Read the model definition and answer for the solid it produces. Units are mm, in the model's axes. Face numbers are marked on the shaded views. A direction names the side the tool comes from. Give positions to 0.01 mm unless a question says otherwise; leave off trailing zeros. Order: outer loops, then holes, each group sorted by start corner. A loop starts at its lowest first (then second) coordinate and runs counter-clockwise, first axis right, second up. Notation, with made-up numbers: (40.5, -18) - (55.5, -18) arc R30 ccw to (55.5, 12) - close; hole circle Ø4 at (-20.75, 79). An arc over 180 degrees is marked (long way). One line per item, written item: value. Start each with the question number.
```python
from build123d import *

# Parameters (mm, degrees)
F0_W     = 105
F0_H     = 90
F0_W_2   = 90
F0_H_2   = 80
F1_DEPTH = 15.3
F2_R     = 5.069848481
F0_W_3   = 69
F0_H_3   = 58
F3_DEPTH = 5.5
F4_DEPTH = 11.8
F5_R     = 4.8284271247


with BuildPart() as f1:
    # F0 (on Top) → F1 (new body, symmetric)
    with BuildSketch(Plane.XY):
        Rectangle(F0_W, F0_H)
        Rectangle(F0_W_2, F0_H_2, mode=Mode.SUBTRACT)
    extrude(amount=F1_DEPTH, both=True)

    # F2
    f2_edges = [f1.edges().sort_by_distance(p)[0] for p in [
        (52.5, -45, 0),
        (-52.5, -45, 0),
        (-52.5, 45, 0),
        (52.5, 45, 0),
    ]]
    fillet(f2_edges, radius=F2_R)

    # F0 (on Top) → F3 (join)
    with BuildSketch(Plane.XY):
        Rectangle(F0_W_2, F0_H_2)
        Rectangle(F0_W_3, F0_H_3, mode=Mode.SUBTRACT)
    extrude(amount=F3_DEPTH)

    # F0 (on Top) → F4 (join)
    with BuildSketch(Plane.XY):
        Rectangle(F0_W_3, F0_H_3)
    extrude(amount=F4_DEPTH)

    # F5
    f5_edges = [f1.edges().sort_by_distance(p)[0] for p in [
        (34.5, -29, 8.65),
        (34.5, 29, 8.65),
        (-34.5, 29, 8.65),
        (-34.5, -29, 8.65),
    ]]
    fillet(f5_edges, radius=F5_R)


solid = f1.part
```
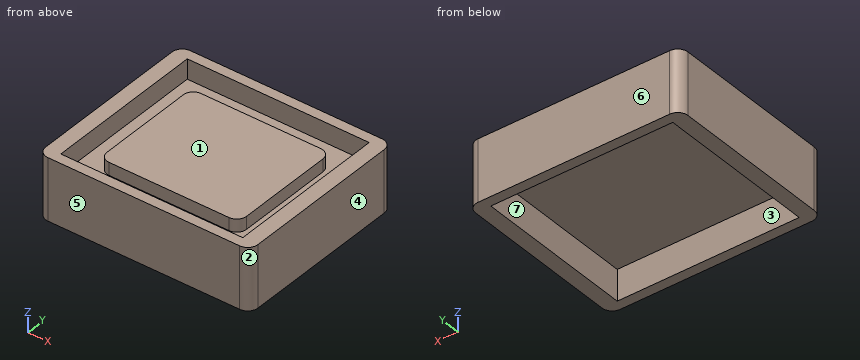
1) Section A-A on z = 9.5 is taken. Write down the section's boundary in (x, y), plus the area to 3 significant figures.
2) Section C-C on y = 7.5 is taken. Write down the section's boundary in (x, z), plus the area to 3 significant figures.
3) Section D-D on x = -23 is taken. Write down the section's boundary in (y, z), plus the area to 3 significant figures.
4) Find the intervals of material crossed by probe 1 along Y at (x, z) = (-10.5, 10.5); probe 2 along X at (y, z) = (-12.5, -10.5); probe 3 along Y at (x, z) = (32, 10.5), in increasing order. Write a range as from..to.
5) For the marked faces 1, 2 and 3, determine the directions among +Z, -Z, +X, -X, +Y, -Y from which every point of the face is accessible in a straight line to the end or side of a thin tool.
6) Each of these flat-tipped pins is pushed along its axis until it touches: pin 1 (1.5 mm diameter, centred on x = -9.5, y = 35, fed in from +Z); pin 2 (12 mm diameter, centred on x = -25.5, y = -27.5, fed in from -Z); pin 3 (17.5 mm diameter, centred on x = -15, y = -3, fed in from +Z). Where does it stop, or does it pass through?
7) Section B-B on x = 40 is taken. Write down the section's boundary in (y, z).
8) The mould has two halves that part along Y. Classify the marked faces 4, 5, 6 and 7: +Y half, -Y half, draft (parallel to the pull), parting line (faces both ways), or undercut.
Solved:
1. outline: (-52.5, -39.93) arc R5.07 ccw to (-47.43, -45) - (47.43, -45) arc R5.07 ccw to (52.5, -39.93) - (52.5, 39.93) arc R5.07 ccw to (47.43, 45) - (-47.43, 45) arc R5.07 ccw to (-52.5, 39.93) - close; (-34.5, -24.17) arc R4.83 ccw to (-29.67, -29) - (29.67, -29) arc R4.83 ccw to (34.5, -24.17) - (34.5, 24.17) arc R4.83 ccw to (29.67, 29) - (-29.67, 29) arc R4.83 ccw to (-34.5, 24.17) - close; hole (-45, -40) - (45, -40) - (45, 40) - (-45, 40) - close
1. area: 6,210 mm2
2. outline: (-52.5, -15.3) - (-45, -15.3) - (-45, 0) - (45, 0) - (45, -15.3) - (52.5, -15.3) - (52.5, 15.3) - (45, 15.3) - (45, 5.5) - (34.5, 5.5) - (34.5, 11.8) - (-34.5, 11.8) - (-34.5, 5.5) - (-45, 5.5) - (-45, 15.3) - (-52.5, 15.3) - close
2. area: 1,390 mm2
3. outline: (-45, -15.3) - (-40, -15.3) - (-40, 0) - (40, 0) - (40, -15.3) - (45, -15.3) - (45, 15.3) - (40, 15.3) - (40, 5.5) - (29, 5.5) - (29, 11.8) - (-29, 11.8) - (-29, 5.5) - (-40, 5.5) - (-40, 15.3) - (-45, 15.3) - close
3. area: 1,110 mm2
4. probe 1: y = -45..-40, -29..29, 40..45
4. probe 2: x = -52.5..-45, 45..52.5
4. probe 3: y = -45..-40, -28.4..28.4, 40..45
5. face 1: +Z
5. face 2: +Z, -Z, +X, -Y
5. face 3: -Z
6. pin 1: stops at z = 5.5
6. pin 2: stops at z = 0
6. pin 3: stops at z = 11.8
7. outline: (-45, -15.3) - (-40, -15.3) - (-40, 0) - (40, 0) - (40, -15.3) - (45, -15.3) - (45, 15.3) - (40, 15.3) - (40, 5.5) - (-40, 5.5) - (-40, 15.3) - (-45, 15.3) - close
8. face 4: draft
8. face 5: -Y half
8. face 6: +Y half
8. face 7: undercut
